Part model, mm, in its own coordinate system. Face numbers are marked on the shaded views. Coordinates: 2 decimals unless noted, no trailing zeros. Loops run counter-clockwise (first coordinate to the right, second up) from the corner with the lowest first, then second, coordinate; pieces in that order, holes last. Notation, with made-up numbers: M 63,20.5 L 105,20.5 A18 cw 105,51.5 Z; hole C -38,-16 d9. An arc over 180 degrees is marked long. Use a Markdown table: item, result. Add a question column.
1) Pin check, flat tip, straight feed: pin 1 Ø6 at (y, z) = (-246.5, 7.5) entering from -X. Stop position of the tip, or through.
2) Band-saw the part on A-A (z = 10.25). List the corners of the cut face in (x, y), plus the area to 3 significant figures.
3) Wall check: probe 1 along Y at (x, z) = (103.5, 1.5); probe 2 along X at (y, z) = (-193, 1); probe 3 along X at (y, z) = (-13, 1.25). Give the ranges that are in metal, low to high. Write a range as from..to.
4) Pull direction Z, two halves, no side cores. Call the marked faces 1 and 2: released by +Z, released by -Z, zero draft, split by the parting line, or undercut.
from build123d import *

# Parameters (mm, degrees)
F0_W     = 355.6
F0_H     = 304.8
F1_DEPTH = 12.7
F2_R     = 6.35
F5_W     = 6.35
F5_H     = 2.032


with BuildPart() as f1:
    # F0 (on Top) → F1 (new body)
    with BuildSketch(Plane.XY):
        with Locations((177.8, -152.4)):
            Rectangle(F0_W, F0_H)
    extrude(amount=F1_DEPTH)

    # F2
    f2_edges = [f1.edges().sort_by_distance(p)[0] for p in [
        (0, -152.4, 12.7),
        (177.8, -304.8, 12.7),
        (355.6, -152.4, 12.7),
        (177.8, 0, 12.7),
    ]]
    fillet(f2_edges, radius=F2_R)

    # F6: sweep along a path in F3
    with BuildLine(Plane(origin=(0, 0, 0), x_dir=(1, 0, 0), z_dir=(0, 0, -1))) as f6_path:
        Line((12.7, 292.1), (12.7, 12.7))
        Line((12.7, 12.7), (342.9, 12.7))
        Line((342.9, 12.7), (342.9, 292.1))
        Line((342.9, 292.1), (12.7, 292.1))
    # F5 (on plane+point) → F6 (sweep, cut)
    with BuildSketch(Plane.XZ.offset(12.7)):
        with Locations((15.875, 1.016)):
            Rectangle(F5_W, F5_H)
    sweep(path=f6_path.line, transition=Transition.RIGHT, mode=Mode.SUBTRACT)


solid = f1.part
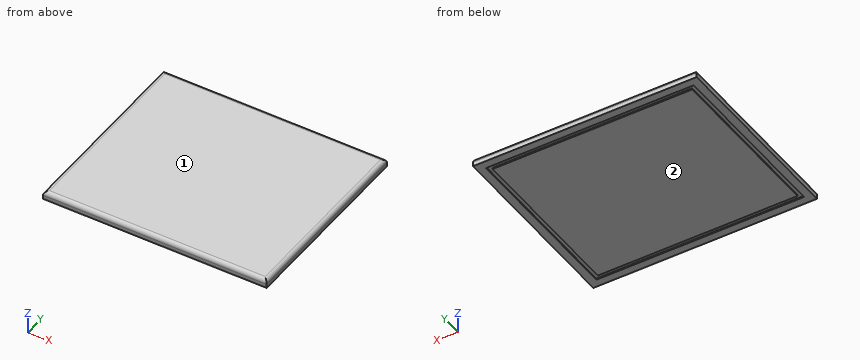
Entries:
| question | item | result |
|---|---|---|
| 1 | pin 1 | x = 0 |
| 2 | outline | M 1.34,-303.46 L 354.26,-303.46 L 354.26,-1.34 L 1.34,-1.34 Z |
| 2 | area | 107,000 mm2 |
| 3 | probe 1 | -304.8..-292.1, -285.75..-19.05, -12.7..0 |
| 3 | probe 2 | 0..12.7, 19.05..336.55, 342.9..355.6 |
| 3 | probe 3 | 0..12.7, 342.9..355.6 |
| 4 | face 1 | released by +Z |
| 4 | face 2 | released by -Z |
